Could you check a few things on this model? Use its own coordinates, in mm. Face numbers are marked on the shaded views. A direction names the side the tool comes from. Coordinates: 2 decimals unless noted, no trailing zeros. Loops run counter-clockwise (first coordinate to the right, second up) from the corner with the lowest first, then second, coordinate; pieces in that order, holes last. Notation, with made-up numbers: (84.5, 39.25) -> (98.5, 39.25) arc R8 ccw to (98.5, 46.25) -> close; hole circle Ø7 at (-39.5, -35). An arc over 180 degrees is marked (long way). One line per question, with ' | ' between items.
Autodesk Inventor part; units mm, degrees
ref_plane "YZ Plane" through (0, 0, 0) normal (1, 0, 0) x (0, 1, 0)
ref_plane "XZ Plane" through (0, 0, 0) normal (0, 1, 0) x (-1, 0, 0)
ref_plane "XY Plane" through (0, 0, 0) normal (0, 0, 1) x (1, 0, 0)
sketch "Sketch1" plane through (0, 0, 0) normal (0, 1, 0) x (-1, 0, 0)
  line L0 (14, -12.5) -> (29, -12.5)
  line L1 (29, -12.5) -> (29, 12.5)
  line L2 (-29, 12.5) -> (-29, -12.5)
  line L3 (-29, -12.5) -> (-14, -12.5)
  line L4 (-14, -12.5) -> (-14, -5.5)
  line L5 (-14, -5.5) -> (14, -5.5)
  line L6 (14, -5.5) -> (14, -12.5)
  line L7 (29, 12.5) -> (-29, 12.5)
  point P0 (0, 0)
  point P1 (-29, 0)
  point P2 (0, -5.5)
  dimension "d0" = 28
  dimension "d1" = 15
  dimension "d2" = 7
  dimension "d3" = 25
extrude "Extrusion1" add sketch "Sketch1" along normal blind 15
sketch "Sketch2" plane through (-29, 0, 12.5) normal (0, 0, 1) x (1, 0, 0)
  line L0 (0, 0) -> (58, 0)
  line L1 (58, 0) -> (58, 15)
  line L2 (0, 15) -> (58, 15)
  line L3 (0, 0) -> (0, 15)
  point P0 (29, 0)
  point P1 (4, 10)
  point P2 (54, 10)
  dimension "d6" = 4
  dimension "d7" = 4
  dimension "d8" = 10
hole "Hole1" at (-25, 10, 12.5) at (25, 10, 12.5) direction (0, 0, -1) diameter 4.5 end through all
sketch "Sketch3" plane through (-29, 0, 12.5) normal (0, 0, 1) x (1, 0, 0)
  circle A0 centre (54, 10) radius 2.25
  circle A1 centre (4, 10) radius 2.25
  line L0 (0, 0) -> (58, 0)
  line L1 (58, 0) -> (58, 15)
  line L2 (0, 15) -> (58, 15)
  line L3 (0, 0) -> (0, 15)
  line L4 (12, 15) -> (12, 3)
  line L5 (12, 3) -> (0, 3)
  line L6 (58, 15) -> (43, 15)
  line L7 (46, 15) -> (46, 3)
  line L8 (46, 3) -> (58, 3)
  point P0 (29, 0)
  point P1 (15, 15)
  dimension "d16" = 3
  dimension "d17" = 3
  dimension "d18" = 3
extrude "Extrusion2" cut sketch "Sketch3" against normal blind 22 contours L3 L2 L4 L5 | L8 L7 L2 L1
sketch "Sketch4" plane through (0, 15, 0) normal (0, 1, 0) x (1, 0, 0)
  circle A0 centre (0, -4.5) radius 5
  line L0 (14, 5.5) -> (-14, 5.5)
  point P0 (0, 0)
  dimension "d21" = 10
  dimension "d22" = 10
extrude "Extrusion3" cut sketch "Sketch4" against normal through all
sketch "Sketch5" plane through (0, 15, 0) normal (0, 1, 0) x (1, 0, 0)
  circle A0 centre (0, -4.5) radius 5
  circle A1 centre (0, -4.5) radius 8
  line L0 (-8, -4.5) -> (-17, -4.5)
  line L1 (-17, -4.5) -> (-29, 4.5)
  line L2 (-29, 12.5) -> (-29, -12.5)
  line L3 (8, -4.5) -> (17, -4.5)
  line L4 (17, -12.5) -> (17, 9.5)
  line L5 (17, -4.5) -> (29, 4.5)
  line L6 (29, -12.5) -> (29, 12.5)
  line L7 (17, 9.5) -> (29, 9.5)
  line L8 (-29, 9.5) -> (-17, 9.5)
  line L9 (-17, -12.5) -> (17, -12.5)
  line L10 (-17, -12.5) -> (-29, -12.5)
  line L11 (-17, -12.5) -> (-17, 9.5)
  line L12 (-17, 9.5) -> (-29, 9.5)
  line L13 (-29, -12.5) -> (-29, 9.5)
  line L14 (29, -12.5) -> (17, -12.5)
  line L15 (29, 9.5) -> (29, -12.5)
  line L16 (29, 9.5) -> (17, 9.5)
  line L17 (17, -12.5) -> (17, 9.5)
  point P0 (0, 0)
  point P1 (-29, -12.5)
  point P2 (0, -12.5)
  dimension "d25" = 3
  dimension "d26" = 5
  dimension "d27" = 5
  dimension "d28" = 8
  dimension "d29" = 8
extrude "Extrusion4" cut sketch "Sketch5" against normal through all contours L3 L4 L9 A1 | A1 L9 L11 L0 | L5 L6 L14 L4 | L11 L10 L2 L1
sketch "Sketch6" plane through (0, 0, 0) normal (0, 0, 1) x (1, 0, 0)
  line L0 (17, 3) -> (17, 15)
  point P0 (0, 0)
  point P1 (0, 9)
  point P2 (17, 9)
hole "Hole2" at (0, 9, 0) direction (0, 0, 1) diameter 4 end through all
equation "\"d27\" = d26"
equation "\"d29\" = d28"
properties part number "Pen Holder"
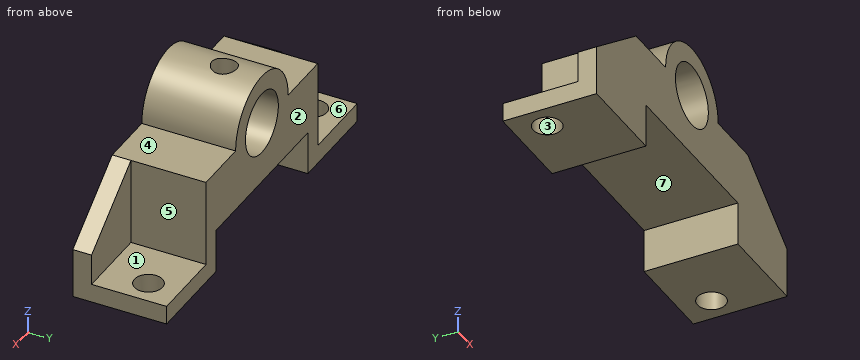
1) On a 3-axis mill with a long thin cutter (end or side, diameter ignored), from which of +Z, -Z, +X, -X, +Y, -Y can I reach the whole of each face in a straight line? I mean the marked faces 4, 5, 6 and 7. Say none if no direction works.
Data:
face 4: +Z, +X, +Y, -Y | face 5: +Z, +X, +Y | face 6: +Z, -X, +Y | face 7: -Z, +Y, -Y
2) If we section it at C-C on x = 0: Please give me the cut outline in (y, z), and give its area (3 significant figures).
Data:
outline: (0, -5.5) -> (15, -5.5) -> (15, -0.5) -> (0, -0.5) -> close; (0, 9.5) -> (7, 9.5) -> (7, 12.5) -> (0, 12.5) -> close; (11, 9.5) -> (15, 9.5) -> (15, 12.5) -> (11, 12.5) -> close | area: 108 mm²
3) If we section it at B-B on y = 4.25: Please give me the cut outline in (x, z), and give its area (3 significant figures).
Data:
outline: (-29, -12.5) -> (-14, -12.5) -> (-14, -5.5) -> (14, -5.5) -> (14, -12.5) -> (29, -12.5) -> (29, -9.5) -> (17, -9.5) -> (17, 4.5) -> (8, 4.5) arc R8 ccw to (-8, 4.5) -> (-17, 4.5) -> (-17, -9.5) -> (-29, -9.5) -> close; hole circle Ø10 at (0, 4.5) | area: 476 mm²
4) I'm going to push flat-ended pins straight in: pin 1 Ø2.5 at (x, y) = (25, 10) entering from +Z; pin 2 Ø9.5 at (x, z) = (-24.5, -5.5) entering from +Y; pin 3 Ø3.5 at (x, y) = (-21.5, 9) entering from +Z; pin 4 Ø1.5 at (x, y) = (5.5, 9) entering from +Z. Where does each tip first touch, or does it pass through?
Data:
pin 1: through | pin 2: y = 15 | pin 3: z = -9.5 | pin 4: z = 10.94
5) We'd pull the mould along Y, two halves only. Please class the marked faces 1, 2 and 3: pulls with the +Y half, pulls with the -Y half, needs draft (parallel to the pull), parting line crosses it, or undercut.
Data:
face 1: needs draft | face 2: pulls with the +Y half | face 3: undercut
6) If we section it at D-D on z = 8.25: Please give me the cut outline in (x, y), and give its area (3 significant figures).
Data:
outline: (-7.07, 0) -> (-3.31, 0) -> (-3.31, 15) -> (-7.07, 15) -> close; (3.31, 0) -> (7.07, 0) -> (7.07, 15) -> (3.31, 15) -> close | area: 113 mm²
7) I need wall thicknesses on line 1 along X through (y, z) = (10, -11.1); line 2 along Y through (x, z) = (-25, -11.55); line 3 along X through (y, z) = (5.5, -9.25). Which ranges of each line are inside material? Lowest first, please. Write a range as from..to.
Data:
line 1: -29..-27.25, -22.75..-14, 14..22.75, 27.25..29 | line 2: 0..7.75, 12.25..15 | line 3: -17..-14, 14..17
8) If we section it at A-A on x = -25: Please give me the cut outline in (y, z), and give its area (3 significant figures).
Data:
outline: (0, -12.5) -> (7.75, -12.5) -> (7.75, -9.5) -> (3, -9.5) -> (3, -1.5) -> (0, -1.5) -> close; (12.25, -12.5) -> (15, -12.5) -> (15, -9.5) -> (12.25, -9.5) -> close | area: 55.5 mm²
